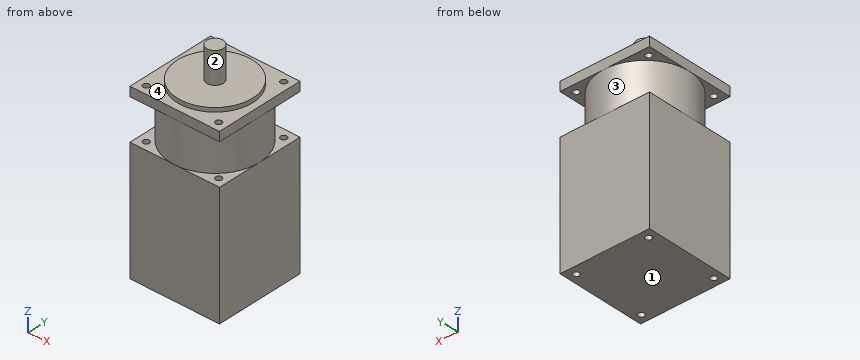
from build123d import *

# Parameters (mm, degrees)
SKETCH_1_W      = 86
SKETCH_1_H      = 86
SKETCH_1_R      = 3
EXTRUDE_1_DEPTH = 118
SKETCH_2_R      = 43
EXTRUDE_2_DEPTH = 39.333333333
SKETCH_3_W      = 86
SKETCH_3_H      = 86
SKETCH_3_R      = 3
EXTRUDE_3_DEPTH = 9
SKETCH_4_R      = 36.25
EXTRUDE_4_DEPTH = 4
SKETCH_5_R      = 8
EXTRUDE_5_DEPTH = 30


with BuildPart() as part:
    # 草图1 → 凸台-拉伸1 (new body)
    with BuildSketch(Plane.XY):
        Rectangle(SKETCH_1_W, SKETCH_1_H)
        with Locations((-34.8, 34.8)):
            Circle(SKETCH_1_R, mode=Mode.SUBTRACT)
        with Locations((34.8, 34.8)):
            Circle(SKETCH_1_R, mode=Mode.SUBTRACT)
        with Locations((34.8, -34.8)):
            Circle(SKETCH_1_R, mode=Mode.SUBTRACT)
        with Locations((-34.8, -34.8)):
            Circle(SKETCH_1_R, mode=Mode.SUBTRACT)
    extrude(amount=EXTRUDE_1_DEPTH)

    # 草图2 → 凸台-拉伸2 (add)
    with BuildSketch(Plane.XY.offset(118)):
        Circle(SKETCH_2_R)
    extrude(amount=EXTRUDE_2_DEPTH)

    # 草图3 → 凸台-拉伸3 (add)
    with BuildSketch(Plane.XY.offset(157.333333333)):
        Rectangle(SKETCH_3_W, SKETCH_3_H)
        with Locations((-34.8, 34.8)):
            Circle(SKETCH_3_R, mode=Mode.SUBTRACT)
        with Locations((34.8, 34.8)):
            Circle(SKETCH_3_R, mode=Mode.SUBTRACT)
        with Locations((34.8, -34.8)):
            Circle(SKETCH_3_R, mode=Mode.SUBTRACT)
        with Locations((-34.8, -34.8)):
            Circle(SKETCH_3_R, mode=Mode.SUBTRACT)
    extrude(amount=EXTRUDE_3_DEPTH)

    # 草图4 → 凸台-拉伸4 (add)
    with BuildSketch(Plane.XY.offset(166.333333333)):
        Circle(SKETCH_4_R)
    extrude(amount=EXTRUDE_4_DEPTH)

    # 草图5 → 凸台-拉伸5 (add)
    with BuildSketch(Plane.XY.offset(170.333333333)):
        Circle(SKETCH_5_R)
    extrude(amount=EXTRUDE_5_DEPTH)


solid = part.part
Geometry check sheet. Reference: the model listing, model coordinates, mm. Face numbers are marked on the shaded views. Round coordinates to 2 decimals unless told otherwise and drop trailing zeros. Write each loop counter-clockwise with the first axis right and the second up, starting at its lowest first coordinate (ties: lowest second). Pieces come first, ordered by that corner, then holes. Notation, with made-up numbers: (22.5, 71.5) - (45.5, 71.5) arc R13 cw to (45.5, 93.5) - close; hole circle Ø11 at (76.5, 41). An arc over 180 degrees is marked (long way). One line per item, written item: value.
1. Cross-section at A-A on z = 13. Record the boundary of the cut face in (x, y).
The answers:
outline: (-43, -43) - (43, -43) - (43, 43) - (-43, 43) - close; hole circle Ø6 at (-34.8, -34.8); hole circle Ø6 at (-34.8, 34.8); hole circle Ø6 at (34.8, -34.8); hole circle Ø6 at (34.8, 34.8)
2. Scan lines: L1, parallel to Y at x = -34.8, z = 163.5; L2, parallel to X at y = -34, z = 46; L3, parallel to Z at x = 17, y = 36.5. Record each from-to range of solid material in increasing order.
The answers:
L1: y = -43 to -37.8, -31.8 to 31.8, 37.8 to 43
L2: x = -43 to -37.69, -31.91 to 31.91, 37.69 to 43
L3: z = 0 to 166.33
3. Mould release check, pull along Z, two halves, no side actions. Record for the marked faces 1, 2, 3 and 4: released by +Z, released by -Z, zero draft, split by the parting line, or undercut.
The answers:
face 1: released by -Z
face 2: zero draft
face 3: undercut
face 4: released by +Z
4. Cross-section at C-C on x = 20.5. Record the boundary of the cut face in (y, z).
The answers:
outline: (-43, 0) - (43, 0) - (43, 118) - (37.8, 118) - (37.8, 157.33) - (43, 157.33) - (43, 166.33) - (29.9, 166.33) - (29.9, 170.33) - (-29.9, 170.33) - (-29.9, 166.33) - (-43, 166.33) - (-43, 157.33) - (-37.8, 157.33) - (-37.8, 118) - (-43, 118) - close
5. Depth check by flat-ended pin: pin 1 Ø5 at (x, y) = (34.8, -34.8) entering from +Z; pin 2 Ø7 at (x, y) = (-34.8, 34.8) entering from -Z; pin 3 Ø8 at (x, y) = (34.8, -34.8) entering from +Z; pin 4 Ø13 at (x, y) = (17.5, 31) entering from +Z. Enter the tip coordinate at first touch or a pass-through.
The answers:
pin 1: passes through
pin 2: stops at z = 0
pin 3: stops at z = 166.33
pin 4: stops at z = 170.33
6. Cross-section at B-B on y = 12. Record the boundary of the cut face in (x, z).
The answers:
outline: (-43, 0) - (43, 0) - (43, 118) - (41.29, 118) - (41.29, 157.33) - (43, 157.33) - (43, 166.33) - (34.21, 166.33) - (34.21, 170.33) - (-34.21, 170.33) - (-34.21, 166.33) - (-43, 166.33) - (-43, 157.33) - (-41.29, 157.33) - (-41.29, 118) - (-43, 118) - close
